Verification items for the finished model (mm, model axes). A direction names the side the tool comes from. Round coordinates to 2 decimals unless told otherwise and drop trailing zeros. Write each loop counter-clockwise with the first axis right and the second up, starting at its lowest first coordinate (ties: lowest second). Pieces come first, ordered by that corner, then holes. Notation, with made-up numbers: (-31.5, -20) -> (-21.5, -20) arc R25 cw to (-21.5, 2) -> close; hole circle Ø2 at (-18, -35). An arc over 180 degrees is marked (long way). Use CSV: the item, a comma, the result in double quotes.
```python
from build123d import *

# Parameters (mm, degrees)
SKETCH1_W           = 8.1
SKETCH1_H           = 4
BOSS_EXTRUDE1_DEPTH = 4
SKETCH2_R           = 1.25
CUT_EXTRUDE1_DEPTH  = 9
SKETCH4_W           = 8.1
SKETCH4_H           = 17.5
BOSS_EXTRUDE2_DEPTH = 2


with BuildPart() as part:
    # Sketch1 → Boss-Extrude1 (new body)
    with BuildSketch(Plane(origin=(0, 0, 0), x_dir=(1, 0, 0), z_dir=(0, 1, 0))):
        with Locations((4.05, 2)):
            Rectangle(SKETCH1_W, SKETCH1_H)
    extrude(amount=BOSS_EXTRUDE1_DEPTH)

    # Sketch2 → Cut-Extrude1 (cut)
    with BuildSketch(Plane(origin=(8.1, 0, 0), x_dir=(0, 0, -1), z_dir=(1, 0, 0))):
        with Locations((2, 2)):
            Circle(SKETCH2_R)
    extrude(amount=-CUT_EXTRUDE1_DEPTH, mode=Mode.SUBTRACT)

    # Sketch4 → Boss-Extrude2 (add)
    with BuildSketch(Plane(origin=(0, 0, 0), x_dir=(-1, 0, 0), z_dir=(0, -1, 0))):
        with Locations((-4.05, 12.75)):
            Rectangle(SKETCH4_W, SKETCH4_H)
    extrude(amount=-BOSS_EXTRUDE2_DEPTH)


solid = part.part
```
Q1. Section check B-B (x = 4.5). Record the cut outline in (y, z).
Filled in:
outline,"(0, -21.5) -> (2, -21.5) -> (2, -4) -> (4, -4) -> (4, 0) -> (0, 0) -> close; hole circle Ø2.5 at (2, -2)"
Q2. Section check C-C (y = 2.8). Record the cut outline in (x, z).
Filled in:
outline,"(0, -4) -> (8.1, -4) -> (8.1, -2.96) -> (0, -2.96) -> close; (0, -1.04) -> (8.1, -1.04) -> (8.1, 0) -> (0, 0) -> close"
Q3. Go/stop test with flat-tipped pins: P1, Ø2, axis at y = 2, z = -2, coming from the -X side; P2, Ø4, axis at x = 2.5, z = -6.5, coming from the +Y side. Record where each tip stops, or that it passes through.
Filled in:
P1,"through"
P2,"y = 2"
Q4. Section check D-D (z = -14.25). Record the cut outline in (x, y), plus the area to 3 significant figures.
Filled in:
outline,"(0, 0) -> (8.1, 0) -> (8.1, 2) -> (0, 2) -> close"
area,"16.2 mm²"
Q5. Access from +Z, -Z, +X, -X, +Y, -Y to the whole of each face (thin tool, end or side, straight path). Record for faces 4 (the flat face through (4, 2, 0)), 5 (the flat face through (4, 3, -4)).
Filled in:
face 4,"+Z, +X, -X, +Y, -Y"
face 5,"-Z, +X, -X, +Y"
Q6. Section check A-A (z = -2). Record the cut outline in (x, y).
Filled in:
outline,"(0, 0) -> (8.1, 0) -> (8.1, 0.75) -> (0, 0.75) -> close; (0, 3.25) -> (8.1, 3.25) -> (8.1, 4) -> (0, 4) -> close"
Q7. Mould release check, pull along Y, two halves, no side actions. Record for faces 1 (the cylindrical face through (4.11, 2.38, -3.19)), 2 (the flat face through (8.1, 1.5, -10.6)), 3 (the flat face through (4, 4, -2)): released by +Y, released by -Y, zero draft, split by the parting line, or undercut.
Filled in:
face 1,"undercut"
face 2,"zero draft"
face 3,"released by +Y"
Q8. Material ranges on L1, parallel to Y at x = 5, z = -2; L2, parallel to Y at x = 6.5, z = -7.25; L3, parallel to Z at x = 4.75, y = 3.1, recorded low to high.
Filled in:
L1,"0 to 0.75, 3.25 to 4"
L2,"0 to 2"
L3,"-4 to -2.59, -1.41 to 0"
